Check sheet for the drawn part. Datum: minimum x, y, z corner. Units: mm. Give positions to 0.01 mm unless a question says otherwise; leave off trailing zeros. Order: outer loops, then holes, each group sorted by start corner. A loop starts at its lowest first (then second) coordinate and runs counter-clockwise, first axis right, second up.
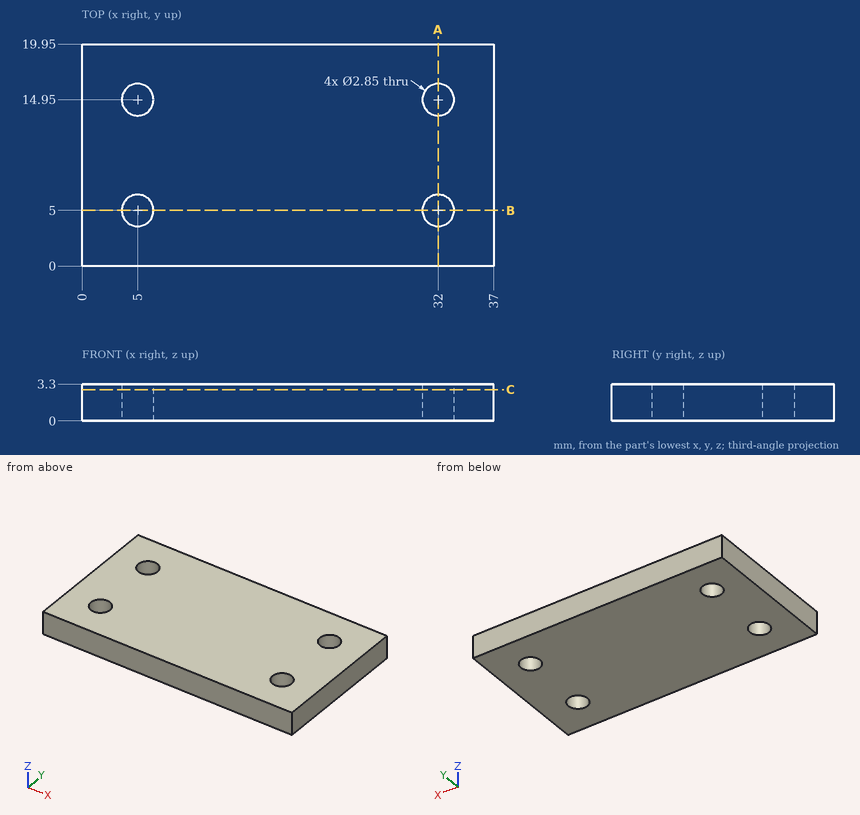
Q1. Sectioned sample at C-C, the plane z = 2.8. Record the cut outline in (x, y) (3 decimals), plus the area to 3 significant figures.
Q2. Sectioned sample at A-A, the plane x = 32. Record the cut outline in (y, z) (3 decimals).
Q3. Sectioned sample at B-B, the plane y = 5. Record the cut outline in (x, z) (3 decimals), plus the area to 3 significant figures.
Q4. Material ranges on line 1 (Y direction, x = 32, z = 1.15) (3 decimals); line 2 (Y direction, x = 31, z = 2.5), recorded low to high.
Filled in:
1. outline: (0, 0) - (37, 0) - (37, 19.95) - (0, 19.95) - close; hole circle Ø2.85 at (5, 5); hole circle Ø2.85 at (5, 14.95); hole circle Ø2.85 at (32, 5); hole circle Ø2.85 at (32, 14.95)
1. area: 713 mm2
2. outline: (0, 0) - (3.575, 0) - (3.575, 3.3) - (0, 3.3) - close; (6.425, 0) - (13.525, 0) - (13.525, 3.3) - (6.425, 3.3) - close; (16.375, 0) - (19.95, 0) - (19.95, 3.3) - (16.375, 3.3) - close
3. outline: (0, 0) - (3.575, 0) - (3.575, 3.3) - (0, 3.3) - close; (6.425, 0) - (30.575, 0) - (30.575, 3.3) - (6.425, 3.3) - close; (33.425, 0) - (37, 0) - (37, 3.3) - (33.425, 3.3) - close
3. area: 103 mm2
4. line 1: y = 0 to 3.575, 6.425 to 13.525, 16.375 to 19.95
4. line 2: y = 0 to 3.98, 6.02 to 13.93, 15.97 to 19.95
